from build123d import *

# Parameters (mm, degrees)
BOSS_EXTRUDE1_DEPTH = 15
SKETCH2_R           = 6.5
BOSS_EXTRUDE2_DEPTH = 22
SKETCH3_R           = 1
BOSS_EXTRUDE3_DEPTH = 3
SKETCH4_W           = 7
SKETCH4_H           = 1
BOSS_EXTRUDE4_DEPTH = 11
SKETCH5_R           = 1.5
BOSS_EXTRUDE5_DEPTH = 20
BOSS_EXTRUDE6_DEPTH = 75
SKETCH7_R           = 1.589398049
BOSS_EXTRUDE7_DEPTH = 50
SKETCH8_R           = 1.5
BOSS_EXTRUDE8_DEPTH = 50
SKETCH9_W           = 7
SKETCH9_H           = 11
BOSS_EXTRUDE9_DEPTH = 50
BOSS_EXTRUDE9_TAPER = -15


with BuildPart() as part:
    # Sketch1 → Boss-Extrude1 (new body)
    with BuildSketch(Plane(origin=(0, 0, 0), x_dir=(1, 0, 0), z_dir=(0, 1, 0))):
        with BuildLine():
            Line((-13, 0), (-13, -21))
            Line((-13, -21), (13, -21))
            Line((13, -21), (13, 0))
            ThreePointArc((13, 0), (0, 13), (-13, 0))
        make_face()
    extrude(amount=BOSS_EXTRUDE1_DEPTH)

    # Sketch2 → Boss-Extrude2 (add)
    with BuildSketch(Plane(origin=(0, 15, 0), x_dir=(1, 0, 0), z_dir=(0, 1, 0))):
        with Locations(Location((0, 0, 0), (0, 0, 270))):
            Circle(SKETCH2_R)
    extrude(amount=BOSS_EXTRUDE2_DEPTH)

    # Sketch3 → Boss-Extrude3 (add)
    with BuildSketch(Plane(origin=(0, 37, 0), x_dir=(1, 0, 0), z_dir=(0, 1, 0))):
        with Locations(Location((0, 0, 0), (0, 0, 270))):
            Circle(SKETCH3_R)
    extrude(amount=BOSS_EXTRUDE3_DEPTH)

    # Sketch4 → Boss-Extrude4 (add)
    with BuildSketch(Plane(origin=(0, 40, 0), x_dir=(1, 0, 0), z_dir=(0, 1, 0))):
        Rectangle(SKETCH4_W, SKETCH4_H)
    extrude(amount=BOSS_EXTRUDE4_DEPTH)

    # Sketch5 → Boss-Extrude5 (add)
    with BuildSketch(Plane.XY.offset(0.5)):
        with Locations(Location((0, 45.870127471, 0), (0, 0, 180))):
            Circle(SKETCH5_R)
    extrude(amount=BOSS_EXTRUDE5_DEPTH)

    # Sketch6 → Boss-Extrude6 (add)
    with BuildSketch(Plane(origin=(0, 0, -0.5), x_dir=(-1, 0, 0), z_dir=(0, 0, -1))):
        with BuildLine():
            Line((1.5, 48.124460967), (1.5, 43.124460967))
            ThreePointArc((1.5, 43.124460967), (0, 41.624460967), (-1.5, 43.124460967))
            Line((-1.5, 43.124460967), (-1.5, 48.124460967))
            ThreePointArc((-1.5, 48.124460967), (0, 49.624460967), (1.5, 48.124460967))
        make_face()
    extrude(amount=BOSS_EXTRUDE6_DEPTH)


with BuildPart() as boss_extrude7_tool:
    # Sketch7 → Boss-Extrude7 (new body)
    with BuildSketch(Plane(origin=(0, 1.929443455, 9.483517563), x_dir=(-1, 0, 0), z_dir=(0, -0.1993679344171976, -0.9799247046208295))):
        with Locations(Location((0, 42.477919634, 0), (0, 0, 160.691778915))):
            Circle(SKETCH7_R)
    extrude(amount=BOSS_EXTRUDE7_DEPTH)


with BuildPart() as part_1:
    add(part.part)


with BuildPart() as part_2:
    # Boss-Extrude7: joined with boss_extrude7_tool
    add(part_1.part.fuse(boss_extrude7_tool.part, tol=0.00001))

    # Sketch8 → Boss-Extrude8 (add)
    with BuildSketch(Plane(origin=(0, 1.687585713, -8.294748783), x_dir=(-1, 0, 0), z_dir=(0, 0.1993679344171843, -0.9799247046208323))):
        with Locations((0, 47.019713669)):
            Circle(SKETCH8_R)
    extrude(amount=BOSS_EXTRUDE8_DEPTH)

    # Sketch9 → Boss-Extrude9 (add)
    with BuildSketch(Plane.XY.offset(0.5)):
        with Locations((0, 45.5)):
            Rectangle(SKETCH9_W, SKETCH9_H)
    extrude(amount=BOSS_EXTRUDE9_DEPTH, taper=BOSS_EXTRUDE9_TAPER)


solid = part_2.part
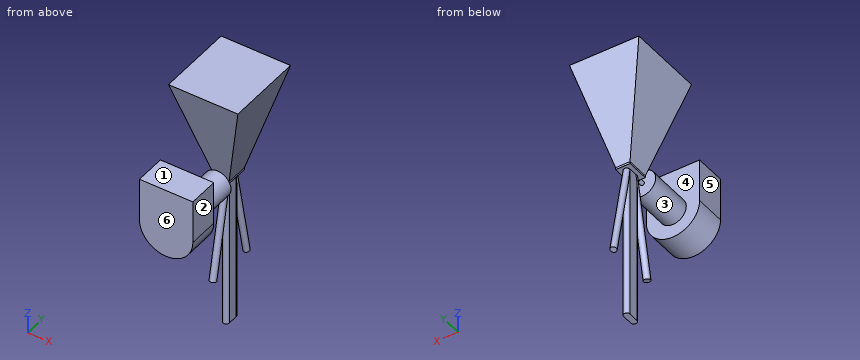
Work out the finished part from the listing and answer in its coordinate system (mm). Face numbers are marked on the shaded views. A direction names the side the tool comes from. Give positions to 0.01 mm unless a question says otherwise; leave off trailing zeros. Write each loop counter-clockwise with the first axis right and the second up, starting at its lowest first coordinate (ties: lowest second). Pieces come first, ordered by that corner, then holes.
Q1. A tool of negligible diameter and unlimited length cuts with its end or side. For the marked faces 1, 2 and 3, from which of +Z, -Z, +X, -X, +Y, -Y can it reach the whole face along a straight path? Write none if from no direction.
Answer:
face 1: +Z, +X, -X, -Y
face 2: +Z, -Z, +X, +Y, -Y
face 3: none
Q2. The part is cut by section B-B on z = -46. State how many separate pieces and enclosed holes the cut face has, and give its area (3 significant figures).
Answer:
separate pieces: 3
enclosed holes: 0
area: 37.4 mm2
Q3. Straight lines are drawn through the part: L1, parallel to Y at x = 1, z = -17; L2, parallel to Y at x = 3, z = -7; L3, parallel to X at y = 13.5, z = 6. For each, find the intervals that lie inside material, in ascending order.
Answer:
L1: y = 38.63 to 41.15, 42.01 to 49.24, 50.3 to 52.58
L2: y = 0 to 15
L3: x = -13 to 13
Q4. The part is cut by section A-A on y = 5.5. Give the vertices of the cut face in (x, z), and give its area (3 significant figures).
Answer:
outline: (-13, 0) arc R13 ccw to (13, 0) - (13, 21) - (-13, 21) - close
area: 811 mm2
Q5. Given pin 1 (5 mm diameter, centred on x = -1, y = 23.5, fed in from -Z); pin 2 (4 mm diameter, centred on y = 45, z = -43.5, fed in from +X); pin 3 (1 mm diameter, centred on y = 25.5, z = 1.5, fed in from +X); pin 4 (1 mm diameter, centred on y = 58, z = 20, fed in from -X), each flat-ended and moving along its own axis, determine where each tip first touches the part or whether it passes through.
Answer:
pin 1: stops at z = -6.5
pin 2: stops at x = 1.5
pin 3: stops at x = 6.42
pin 4: passes through
Q6. For a pull along Y with two mould halves and no side action, classify the marked faces 4, 5 and 6 as released by +Y, released by -Y, zero draft, split by the parting line, or undercut.
Answer:
face 4: undercut
face 5: zero draft
face 6: released by -Y
